```python
from build123d import *

# Parameters (mm, degrees)
EXTRUDE1_DEPTH = 9.525
SKETCH2_R      = 18.135228151
SKETCH2_R_2    = 13.849910733
EXTRUDE2_DEPTH = 9.525
SKETCH5_W      = 21.692133904
SKETCH5_H      = 5.39360198
SKETCH5_W_2    = 5.39360198
SKETCH5_H_2    = 21.692133904
SKETCH5_W_3    = 21.692133903
EXTRUDE4_DEPTH = 6.35


with BuildPart() as part:
    # Sketch1 → Extrude1 (new body)
    with BuildSketch(Plane(origin=(0, 0, 0), x_dir=(1, 0, 0), z_dir=(0, 1, 0))):
        with BuildLine():
            Line((80.952795926, -6.933070377), (3.175, -6.933070377))
            ThreePointArc((3.175, -6.933070377), (0.92993597, -6.003134407), (0, -3.758070377))
            Line((0, -3.758070377), (0, 72.612142843))
            ThreePointArc((0, 72.612142843), (1.339107796, 75.845035046), (4.572, 77.184142843))
            Line((4.572, 77.184142843), (79.555795926, 77.184142843))
            ThreePointArc((79.555795926, 77.184142843), (82.78868813, 75.845035046), (84.127795926, 72.612142843))
            Line((84.127795926, 72.612142843), (84.127795926, -3.758070377))
            ThreePointArc((84.127795926, -3.758070377), (83.197859957, -6.003134407), (80.952795926, -6.933070377))
        make_face()
    extrude(amount=-EXTRUDE1_DEPTH)

    # Sketch2 → Extrude2 (add)
    with BuildSketch(Plane(origin=(0, 0, 0), x_dir=(1, 0, 0), z_dir=(0, 1, 0))):
        with Locations(Location((42.063897963, 35.130827586, 0), (0, 0, 90))):
            Circle(SKETCH2_R)
        with Locations(Location((42.063897963, 35.130827586, 0), (0, 0, 90))):
            Circle(SKETCH2_R_2, mode=Mode.SUBTRACT)
    extrude(amount=EXTRUDE2_DEPTH)

    # Sketch5 → Extrude4 (add)
    with BuildSketch(Plane(origin=(0, 0, 0), x_dir=(1, 0, 0), z_dir=(0, 1, 0))):
        with Locations((70.300158538, 34.427036233)):
            Rectangle(SKETCH5_W, SKETCH5_H)
        with Locations((42.063897963, 6.190775658)):
            Rectangle(SKETCH5_W_2, SKETCH5_H_2)
        with Locations((13.827637389, 34.427036233)):
            Rectangle(SKETCH5_W_3, SKETCH5_H)
        with Locations((42.063897963, 62.663296808)):
            Rectangle(SKETCH5_W_2, SKETCH5_H_2)
    extrude(amount=EXTRUDE4_DEPTH)


solid = part.part
```
Geometry check sheet. Reference: the model listing, model coordinates, mm. A direction names the side the tool comes from. Coordinates: 2 decimals unless noted, no trailing zeros. Loops run counter-clockwise (first coordinate to the right, second up) from the corner with the lowest first, then second, coordinate; pieces in that order, holes last. Notation, with made-up numbers: (19, 84) - (58, 84) arc R19 ccw to (58, 98) - close; hole circle Ø8 at (-37, -28.75). An arc over 180 degrees is marked (long way). One line per item, written item: value. Start each with the question number.
(1) Cross-section at B-B on x = 78. Enter the section's corners in (y, z) (3 decimals), plus the area to 3 significant figures.
(2) Mould release check, pull along X, two halves, no side actions. Record for faces 6 (the cylindrical face through (83.2, -4.7, 6)), 7 (the cylindrical face through (47.368, 4.696, -47.925)), 8 (the flat face through (70, 3, -37.124)): released by +X, released by -X, zero draft, split by the parting line, or undercut.
(3) Depth check by flat-ended pin: P1, Ø4.5, axis at x = 15, z = -33.5, coming from the +Y side; P2, Ø1.6, axis at x = 41.5, y = 3.5, coming from the +Z side; P3, Ø25, axis at x = 42.06, z = -35.13, coming from the +Y side. Enter the tip coordinate at first touch or a pass-through.
(4) Material ranges on line 1 (X direction, y = 4, z = -68.5); line 2 (Y direction, x = 22, z = -34) (3 decimals); line 3 (Y direction, x = 61.5, z = -46) (3 decimals), recorded low to high. Write a range as [from, to].
(5) Cross-section at D-D on z = -29. Enter the section's corners in (x, y) (3 decimals).
(6) Cross-section at A-A on z = -1.5. Enter the section's corners in (x, y) (3 decimals).
(7) Cross-section at C-C on y = 1.5. Enter the section's corners in (x, z).
(8) Tool access check on faces 1 (the flat face through (42, 6.35, -6)), 2 (the flat face through (70, 3, -31.73)), 3 (the flat face through (39.367, 3, -6)), 4 (the flat face through (2.982, 3, -34)), 5 (the flat face through (13, 3, -37.124)). Record the directions out of +Z, -Z, +X, -X, +Y, -Y that give a thin tool (end or side, any length) a straight path to the whole face; none if there is none.
Results below:
1. outline: (-9.525, -77.184) - (0, -77.184) - (0, -37.124) - (6.35, -37.124) - (6.35, -31.73) - (0, -31.73) - (0, 6.933) - (-9.525, 6.933) - close
1. area: 835 mm2
2. face 6: released by +X
2. face 7: undercut
2. face 8: zero draft
3. P1: stops at y = 6.35
3. P2: stops at z = 4.66
3. P3: stops at y = 0
4. line 1: x = [39.37, 44.76]
4. line 2: y = [-9.525, 6.35]
4. line 3: y = [-9.525, 0]
5. outline: (0, -9.525) - (84.128, -9.525) - (84.128, 0) - (59.131, 0) - (59.131, 9.525) - (54.483, 9.525) - (54.483, 0) - (29.645, 0) - (29.645, 9.525) - (24.996, 9.525) - (24.996, 0) - (0, 0) - close
6. outline: (0, -9.525) - (84.128, -9.525) - (84.128, 0) - (44.761, 0) - (44.761, 6.35) - (39.367, 6.35) - (39.367, 0) - (0, 0) - close
7. outline: (2.98, -37.12) - (24.04, -37.12) arc R18.14 ccw to (39.37, -53.06) - (39.37, -73.51) - (44.76, -73.51) - (44.76, -53.06) arc R18.14 ccw to (60.09, -37.12) - (81.15, -37.12) - (81.15, -31.73) - (59.88, -31.73) arc R18.14 ccw to (43.29, -17.04) - (44.76, -17.04) - (44.76, 4.66) - (39.37, 4.66) - (39.37, -17.04) - (40.84, -17.04) arc R18.14 ccw to (24.25, -31.73) - (2.98, -31.73) - close; hole circle Ø27.7 at (42.06, -35.13)
8. face 1: +Z, +X, -X, +Y
8. face 2: +Z, +X, +Y
8. face 3: +Z, -X, +Y
8. face 4: +Z, -Z, -X, +Y
8. face 5: -Z, -X, +Y
